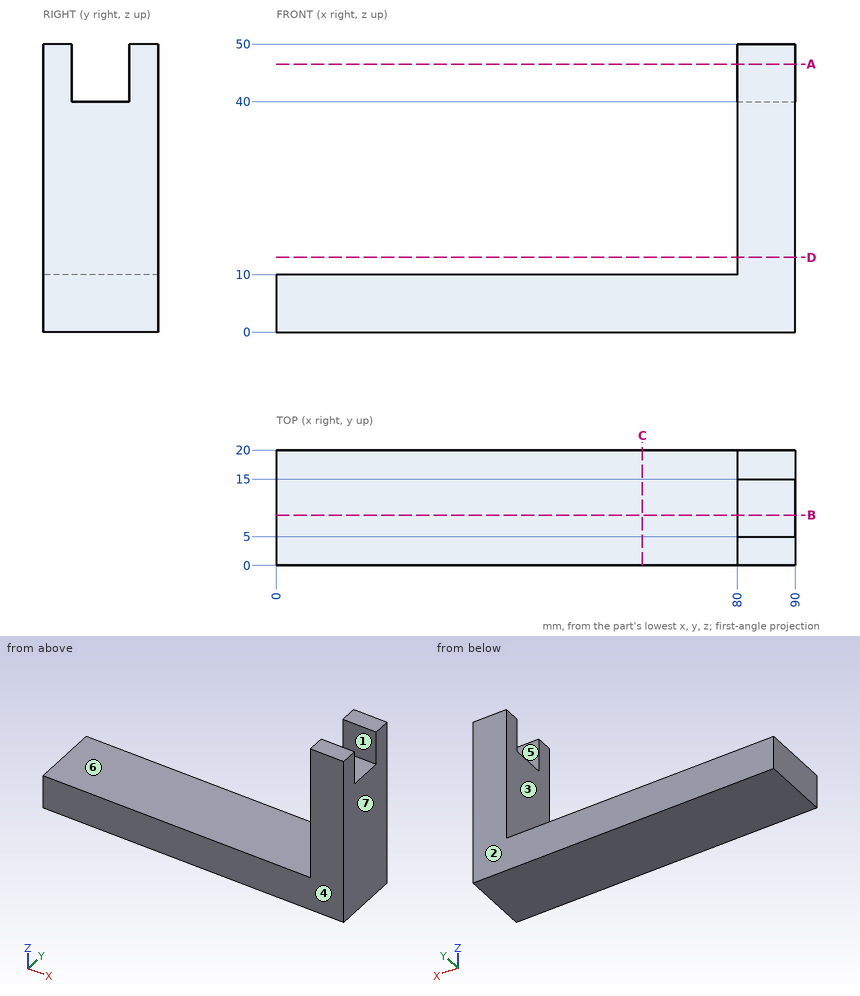
Could you check a few things on this drawing? It's one solid part, dimensions in mm from its lowest x, y, z. A direction names the side the tool comes from. Give positions to 0.01 mm unless a question says otherwise; leave off trailing zeros. Write each loop counter-clockwise with the first axis right and the second up, starting at its lowest first coordinate (ties: lowest second). Pieces come first, ordered by that corner, then holes. Notation, with made-up numbers: (59, -2.75) - (105, -2.75) arc R29 ccw to (105, 19.25) - close; hole circle Ø5 at (25, 46). An arc over 180 degrees is marked (long way). Use CSV: the item, a comma, the result in double quotes. Start each with the question number.
Item 1: I want a section at B-B, the plane y = 8.75. Please give me the cut outline in (x, z), then the cut area to 3 significant figures.
Item 2: I'm going to push a flat-ended pin straight in: pin 1 (3 mm diameter, centred on x = 85, y = 12, fed in from +Z). Where does the tip first touch, or does it pass through?
Item 3: For the marked faces 5, 6 and 7, which set-ups out of +Z, -Z, +X, -X, +Y, -Y let a thin tool reach every point of the face, with its end or its side?
Item 4: I want a section at C-C, the plane x = 63.5. Please give me the cut outline in (y, z), then the cut area to 3 significant figures.
Item 5: If we mould it in two halves opening along Y, with no side actions, what happens to the marked faces 1, 2, 3 and 4? For each: pulls with the +Y half, pulls with the -Y half, needs draft (parallel to the pull), parting line crosses it, or undercut.
Item 6: I want a section at A-A, the plane z = 46.5. Please give me the cut outline in (x, y), then the cut area to 3 significant figures.
Item 7: I want a section at D-D, the plane z = 13. Please give me the cut outline in (x, y), then the cut area to 3 significant figures.
Item 8: If I drill on line 1 along X through (y, z) = (9, 23); line 2 along Z through (x, y) = (52.5, 15), over which ranges is the centre line in solid material (lowest first)?
Findings:
1,outline,"(0, 0) - (90, 0) - (90, 40) - (80, 40) - (80, 10) - (0, 10) - close"
1,area,"1,200 mm2"
2,pin 1,"stops at z = 40"
3,face 5,"+Z, +X, -X"
3,face 6,"+Z, -X, +Y, -Y"
3,face 7,"+Z, -Z, +X, +Y, -Y"
4,outline,"(0, 0) - (20, 0) - (20, 10) - (0, 10) - close"
4,area,"200 mm2"
5,face 1,"undercut"
5,face 2,"pulls with the +Y half"
5,face 3,"needs draft"
5,face 4,"pulls with the -Y half"
6,outline,"(80, 0) - (90, 0) - (90, 5) - (80, 5) - close; (80, 15) - (90, 15) - (90, 20) - (80, 20) - close"
6,area,"100 mm2"
7,outline,"(80, 0) - (90, 0) - (90, 20) - (80, 20) - close"
7,area,"200 mm2"
8,line 1,"x = 80 to 90"
8,line 2,"z = 0 to 10"
